The listing builds one solid part. Answer for the finished solid, in the listing's coordinates (mm). Face numbers are marked on the shaded views. A direction names the side the tool comes from. Coordinates: 2 decimals unless noted, no trailing zeros. Order: outer loops, then holes, each group sorted by start corner. A loop starts at its lowest first (then second) coordinate and runs counter-clockwise, first axis right, second up. Notation, with made-up numbers: (5.5, 9.5) -> (37.5, 9.5) arc R15 cw to (37.5, 38.5) -> close; hole circle Ø10 at (8.5, 67.5). An arc over 180 degrees is marked (long way). One line per question, with ' | ' between items.
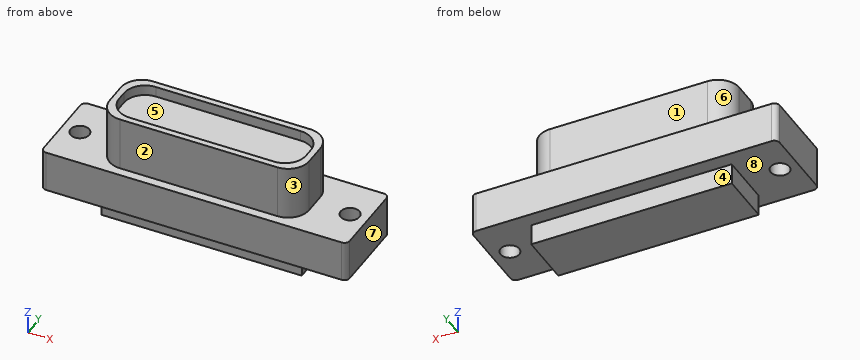
from build123d import *

# Parameters (mm, degrees)
SKETCH1_W                 = 36.83
SKETCH1_H                 = 9.906
BASE_DEPTH                = 4.9784
BOSS_EXTRUDE2_DEPTH       = 6.5024
F_4_40_TAPPED_HOLE1_D     = 2.2606
F_4_40_TAPPED_HOLE1_DEPTH = 7.5946
F_4_40_TAPPED_HOLE1_TIP   = 0.679152758
SKETCH5_W                 = 24.13
SKETCH5_H                 = 6.35
BOSS_EXTRUDE3_DEPTH       = 2.54
CUT_EXTRUDE1_DEPTH        = 1.27
FILLET1_R                 = 0.635


with BuildPart() as part:
    # Sketch1 → Base (new body)
    with BuildSketch(Plane.XY):
        Rectangle(SKETCH1_W, SKETCH1_H)
    extrude(amount=BASE_DEPTH)

    # Sketch2 → Boss-Extrude2 (add)
    with BuildSketch(Plane.XY.offset(4.9784)):
        with BuildLine():
            Line((-9.4742, -3.8608), (9.4742, -3.8608))
            ThreePointArc((9.4742, -3.8608), (11.270251224, -3.116851224), (12.0142, -1.3208))
            Line((12.0142, -1.3208), (12.0142, 1.3208))
            ThreePointArc((12.0142, 1.3208), (11.270251224, 3.116851224), (9.4742, 3.8608))
            Line((9.4742, 3.8608), (-9.4742, 3.8608))
            ThreePointArc((-9.4742, 3.8608), (-11.270251224, 3.116851224), (-12.0142, 1.3208))
            Line((-12.0142, 1.3208), (-12.0142, -1.3208))
            ThreePointArc((-12.0142, -1.3208), (-11.270251224, -3.116851224), (-9.4742, -3.8608))
        make_face()
    extrude(amount=BOSS_EXTRUDE2_DEPTH)

    # #4-40 Tapped Hole1
    with Locations(Plane.XY.offset(4.9784)):
        with Locations((-16.256, 0), (16.256, 0)):
            Hole(F_4_40_TAPPED_HOLE1_D / 2, depth=F_4_40_TAPPED_HOLE1_DEPTH)
            with Locations((0, 0, -(F_4_40_TAPPED_HOLE1_DEPTH + F_4_40_TAPPED_HOLE1_TIP / 2))):  # 118° drill point
                Cone(0, F_4_40_TAPPED_HOLE1_D / 2, F_4_40_TAPPED_HOLE1_TIP, mode=Mode.SUBTRACT)

    # Sketch5 → Boss-Extrude3 (add)
    with BuildSketch(Plane(origin=(0, 0, 0), x_dir=(-1, 0, 0), z_dir=(0, 0, -1))):
        Rectangle(SKETCH5_W, SKETCH5_H)
    extrude(amount=BOSS_EXTRUDE3_DEPTH)

    # Sketch6 → Cut-Extrude1 (cut)
    with BuildSketch(Plane.XY.offset(11.4808)):
        with BuildLine():
            Line((-8.7122, -3.0988), (8.7122, -3.0988))
            ThreePointArc((8.7122, -3.0988), (10.508251224, -2.354851224), (11.2522, -0.5588))
            Line((11.2522, -0.5588), (11.2522, 0.5588))
            ThreePointArc((11.2522, 0.5588), (10.508251224, 2.354851224), (8.7122, 3.0988))
            Line((8.7122, 3.0988), (-8.7122, 3.0988))
            ThreePointArc((-8.7122, 3.0988), (-10.508251224, 2.354851224), (-11.2522, 0.5588))
            Line((-11.2522, 0.5588), (-11.2522, -0.5588))
            ThreePointArc((-11.2522, -0.5588), (-10.508251224, -2.354851224), (-8.7122, -3.0988))
        make_face()
    extrude(amount=-CUT_EXTRUDE1_DEPTH, mode=Mode.SUBTRACT)

    # Fillet1
    fillet1_edges = [part.edges().sort_by_distance(p)[0] for p in [
        (18.415, -4.953, 2.4892),
        (-18.415, -4.953, 2.4892),
        (-18.415, 4.953, 2.4892),
        (18.415, 4.953, 2.4892),
    ]]
    fillet(fillet1_edges, radius=FILLET1_R)


solid = part.part
Item 1: Section D-D, the plane x = -16 is taken. Give the vertices of the cut face in (y, z), plus the area to 3 significant figures.
Computed values:
outline: (-4.95, 0) -> (-1.1, 0) -> (-1.1, 4.98) -> (-4.95, 4.98) -> close; (1.1, 0) -> (4.95, 0) -> (4.95, 4.98) -> (1.1, 4.98) -> close | area: 38.4 mm^2
Item 2: Each of these flat-tipped pins is pushed along its axis until it touches: pin 1 Ø1 at (y, z) = (3.5, 9.5) entering from -X; pin 2 Ø1 at (x, z) = (-2, 11) entering from -Y; pin 3 Ø1.3 at (y, z) = (0.5, 8) entering from +X. Where does it stop, or does it pass through?
Computed values:
pin 1: stops at x = -11.38 | pin 2: stops at y = -3.86 | pin 3: stops at x = 12.01
Item 3: Section C-C, the plane z = 7.5 is taken. Give the vertices of the cut face in (x, y).
Computed values:
outline: (-12.01, -1.32) arc R2.54 ccw to (-9.47, -3.86) -> (9.47, -3.86) arc R2.54 ccw to (12.01, -1.32) -> (12.01, 1.32) arc R2.54 ccw to (9.47, 3.86) -> (-9.47, 3.86) arc R2.54 ccw to (-12.01, 1.32) -> close
Item 4: Section A-A, the plane y = 0 is taken. Give the vertices of the cut face in (x, z) (3 decimals), plus the area to 3 significant figures.
Computed values:
outline: (-18.415, 0) -> (-17.386, 0) -> (-17.386, 4.978) -> (-18.415, 4.978) -> close; (-15.126, 0) -> (-12.065, 0) -> (-12.065, -2.54) -> (12.065, -2.54) -> (12.065, 0) -> (15.126, 0) -> (15.126, 4.978) -> (12.014, 4.978) -> (12.014, 11.481) -> (11.252, 11.481) -> (11.252, 10.211) -> (-11.252, 10.211) -> (-11.252, 11.481) -> (-12.014, 11.481) -> (-12.014, 4.978) -> (-15.126, 4.978) -> close; (17.386, 0) -> (18.415, 0) -> (18.415, 4.978) -> (17.386, 4.978) -> close | area: 350 mm^2
Item 5: Determine the mould class of the marked faces 5, 6, 7 and 8 for opening direction X: pulls with the +X half, pulls with the -X half, needs draft (parallel to the pull), parting line crosses it, or undercut.
Computed values:
face 5: undercut | face 6: pulls with the -X half | face 7: pulls with the +X half | face 8: needs draft
Item 6: Section B-B, the plane z = 4 is taken. Give the vertices of the cut face in (x, y) (3 decimals).
Computed values:
outline: (-18.415, -4.318) arc R0.635 ccw to (-17.78, -4.953) -> (17.78, -4.953) arc R0.635 ccw to (18.415, -4.318) -> (18.415, 4.318) arc R0.635 ccw to (17.78, 4.953) -> (-17.78, 4.953) arc R0.635 ccw to (-18.415, 4.318) -> close; hole circle Ø2.261 at (-16.256, 0); hole circle Ø2.261 at (16.256, 0)
Item 7: For the marked faces 1, 2, 3 and 4, determine the directions among +Z, -Z, +X, -X, +Y, -Y from which every point of the face is accessible in a straight line to the end or side of a thin tool.
Computed values:
face 1: +Z, +X, -X, +Y | face 2: +Z, +X, -X, -Y | face 3: +Z, +X, -Y | face 4: -Z, +X, -X, +Y
Item 8: Find the intervals of material crossed by L1, parallel to Y at x = 1.5, z = 10.5; L2, parallel to Z at x = -6, y = 0.25; L3, parallel to Z at x = 13, y = -3, in increasing order.
Computed values:
L1: y = -3.86 to -3.1, 3.1 to 3.86 | L2: z = -2.54 to 10.21 | L3: z = 0 to 4.98
